```python
from build123d import *

# Parameters (mm, degrees)
SALIENTE_EXTRUIR1_DEPTH = 130
REDONDEO1_R             = 2
SALIENTE_EXTRUIR2_DEPTH = 120
CROQUIS3_R              = 4.5
CORTAR_EXTRUIR1_DEPTH   = 20
CROQUIS4_W              = 24
CROQUIS4_H              = 24
SALIENTE_EXTRUIR3_DEPTH = 30
CORTAR_EXTRUIR2_DEPTH   = 50


with BuildPart() as part:
    # Croquis1 → Saliente-Extruir1 (new body, symmetric)
    with BuildSketch(Plane.XY):
        Polygon((-12, 12), (0, 12), (0, 15), (-15, 15), (-15, -15), (0, -15), (0, -12), (-12, -12), align=None)
    extrude(amount=SALIENTE_EXTRUIR1_DEPTH, both=True)

    # Redondeo1
    redondeo1_edges = [part.edges().sort_by_distance(p)[0] for p in [
        (-15, 15, 0),
        (-15, -15, 0),
    ]]
    fillet(redondeo1_edges, radius=REDONDEO1_R)

    # Croquis2 → Saliente-Extruir2 (add)
    with BuildSketch(Plane.XY.offset(130)):
        with BuildLine():
            Line((-15, 43), (-15, 17))
            ThreePointArc((-15, 17), (-14.414213562, 15.585786438), (-13, 15))
            Line((-13, 15), (0, 15))
            Line((0, 15), (0, 18))
            Line((0, 18), (-12, 18))
            Line((-12, 18), (-12, 42))
            Line((-12, 42), (0, 42))
            Line((0, 42), (0, 45))
            Line((0, 45), (-13, 45))
            ThreePointArc((-13, 45), (-14.414213562, 44.414213562), (-15, 43))
        make_face()
    extrude(amount=-SALIENTE_EXTRUIR2_DEPTH)

    # Croquis3 → Cortar-Extruir1 (cut)
    with BuildSketch(Plane.ZY.offset(15)):
        with Locations((120, 36)):
            Circle(CROQUIS3_R)
        with Locations((20, 36)):
            Circle(CROQUIS3_R)
    extrude(amount=-CORTAR_EXTRUIR1_DEPTH, mode=Mode.SUBTRACT)

    # Croquis4 → Saliente-Extruir3 (add)
    with BuildSketch(Plane.ZY.offset(15)):
        with BuildLine():
            Line((128, -15), (102, -15))
            ThreePointArc((102, -15), (100.585786438, -14.414213562), (100, -13))
            Line((100, -13), (100, 13))
            ThreePointArc((100, 13), (100.585786438, 14.414213562), (102, 15))
            Line((102, 15), (128, 15))
            ThreePointArc((128, 15), (129.414213562, 14.414213562), (130, 13))
            Line((130, 13), (130, -13))
            ThreePointArc((130, -13), (129.414213562, -14.414213562), (128, -15))
        make_face()
        with Locations((115, 0)):
            Rectangle(CROQUIS4_W, CROQUIS4_H, mode=Mode.SUBTRACT)
    extrude(amount=SALIENTE_EXTRUIR3_DEPTH)

    # Croquis5 → Cortar-Extruir2 (cut)
    with BuildSketch(Plane.XY.offset(130)):
        Polygon((-45, -15), (-15, 15), (-45, 15), align=None)
    extrude(amount=-CORTAR_EXTRUIR2_DEPTH, mode=Mode.SUBTRACT)


solid = part.part
```
CAD build for the part. Positions are in the model's coordinates, mm. A direction names the side the tool comes from. Round coordinates to 2 decimals unless told otherwise and drop trailing zeros. Write each loop counter-clockwise with the first axis right and the second up, starting at its lowest first coordinate (ties: lowest second). Pieces come first, ordered by that corner, then holes. Notation, with made-up numbers: (15.25, 44) - (67.25, 44) arc R19 cw to (67.25, 48) - close; hole circle Ø6 at (73, 36). An arc over 180 degrees is marked (long way). Write item = value, one per line. Start each with the question number.
Q1. Probe L1, parallel to Y at x = -6, z = 63; L2, parallel to Y at x = -2, z = -78.5; L3, parallel to Y at x = -13.9, z = 120. List the from-to ranges inside material, lowest first. Write a range as from..to.
Q2. Which spindle directions (+Z, -Z, +X, -X, +Y, -Y) get a long thin tool onto all of the face, cutting with end or side? Do faces 5 (the flat face through (-15, 0, 115)), 6 (the flat face through (-15, 0, -13)), 7 (the flat face through (-6, 42, 71)), 8 (the flat face through (-13, 30, 10)). Say none if no direction does.
Q3. Band-saw the part on B-B (x = -2.5). Give the cut face in (y, z), then the cut area to 3 significant figures.
Q4. Mould opens along Z. For faces 1 (the flat face through (-18, 4, 130)), 2 (the flat face through (-12, 0, 2)), 3 (the flat face through (-13, 0, -130)), 4 (the flat face through (-28, -12, 115)) say: pulls with the +Z half, pulls with the -Z half, needs draft (parallel to the pull), parting line crosses it, or undercut.
Q5. Band-saw the part on C-C (y = -4.5). Give the cut face in (x, z), then the cut area to 3 significant figures.
Q6. Band-saw the part on D-D (x = -38). Give the cut face in (y, z), then the cut area to 3 significant figures.
Q7. Band-saw the part on A-A (z = 20). Give the cut face in (x, y), then the cut area to 3 significant figures.
Q8. Drop flat-ended pins along their axis: pin 1 (2 mm diameter, centred on x = -5.5, z = -92, fed in from +Y); pin 2 (1 mm diameter, centred on y = 18, z = 98, fed in from -X); pin 3 (13 mm diameter, centred on x = -26, y = 2.5, fed in from -Z); pin 4 (1 mm diameter, centred on y = -14, z = 114.5, fed in from +X). Give the stop position or say it passes through.
Answers below:
q1.L1 = -15..-12, 12..18, 42..45
q1.L2 = -15..-12, 12..15
q1.L3 = -14.79..14.79, 15.21..31.5, 40.5..44.79
q2.face_5 = -X
q2.face_6 = -Z, -X, +Y, -Y
q2.face_7 = +Z, -Z, +X
q2.face_8 = -Z, +X, -X, +Y
q3.outline = (-15, -130) - (-12, -130) - (-12, 130) - (-15, 130) - close; (12, -130) - (15, -130) - (15, 10) - (18, 10) - (18, 130) - (12, 130) - close; (42, 10) - (45, 10) - (45, 130) - (42, 130) - close
q3.area = 2,280 mm2
q4.face_1 = pulls with the +Z half
q4.face_2 = needs draft
q4.face_3 = pulls with the -Z half
q4.face_4 = undercut
q5.outline = (-34.5, 100) - (-15, 100) - (-15, -130) - (-12, -130) - (-12, 130) - (-34.5, 130) - (-34.5, 127) - (-15, 127) - (-15, 103) - (-34.5, 103) - close
q5.area = 897 mm2
q6.outline = (-15, 102) arc R2 ccw to (-13, 100) - (-8, 100) - (-8, 103) - (-12, 103) - (-12, 127) - (-8, 127) - (-8, 130) - (-13, 130) arc R2 ccw to (-15, 128) - close
q6.area = 112 mm2
q7.outline = (-15, -13) arc R2 ccw to (-13, -15) - (0, -15) - (0, -12) - (-12, -12) - (-12, 12) - (0, 12) - (0, 18) - (-12, 18) - (-12, 31.5) - (-15, 31.5) - (-15, 17) arc R2 ccw to (-13, 15) arc R2 ccw to (-15, 13) - close; (-15, 40.5) - (-12, 40.5) - (-12, 42) - (0, 42) - (0, 45) - (-13, 45) arc R2 ccw to (-15, 43) - close
q7.area = 294 mm2
q8.pin_1 = 15
q8.pin_2 = -15
q8.pin_3 = 100
q8.pin_4 = 0
